Could you check a few things on this drawing? It's one solid part, dimensions in mm from its lowest x, y, z. A direction names the side the tool comes from. Coordinates: 2 decimals unless noted, no trailing zeros. Order: outer loops, then holes, each group sorted by start corner. A loop starts at its lowest first (then second) coordinate and runs counter-clockwise, first axis right, second up. Notation, with made-up numbers: (-34.5, 77.5) - (10.5, 77.5) arc R26 cw to (10.5, 100.5) - close; hole circle Ø1 at (46, 26.5). An arc over 180 degrees is marked (long way). Answer in a Markdown table with one row per item. Add a question column.
Item 1: I want a section at D-D (y = 9). Count the separate pieces of the cut face and the enclosed holes in it.
Item 2: On a 3-axis mill with a long thin cutter (end or side, diameter ignored), from which of +Z, -Z, +X, -X, +Y, -Y can I reach the whole of each face in a straight line? I mean the marked faces 4 and 5. Say none if no direction works.
Item 3: I want a section at B-B (x = 15.5). Please give me the cut outline in (y, z).
Item 4: Will these pins go through, and if not, where does the flat tip stop? pin 1 Ø4 at (x, y) = (7, 9) entering from +Z; pin 2 Ø5 at (y, z) = (12.5, 24) entering from +X; pin 3 Ø5 at (x, z) = (31, 7.5) entering from +Y; pin 4 Ø3 at (y, z) = (2.5, 28) entering from +X.
Item 5: I want a section at C-C (z = 21). Please give me the cut outline in (x, y) (1 decimal).
Item 6: Thinking about a two-plate mould opening in X: for the marked faces 1, 2 and 3, which applies, +X half, -X half, draft (parallel to the pull), parting line (faces both ways), or undercut?
Item 7: I want a section at A-A (z = 7). Please give me the cut outline in (x, y).
Item 8: If I drill on line 1 along Z through (x, y) = (24, 4.5); line 2 along X through (y, z) = (16.5, 13); line 3 along Z through (x, y) = (17.5, 2.5), over which ranges is the centre line in solid material (lowest first)? Write a range as from..to.
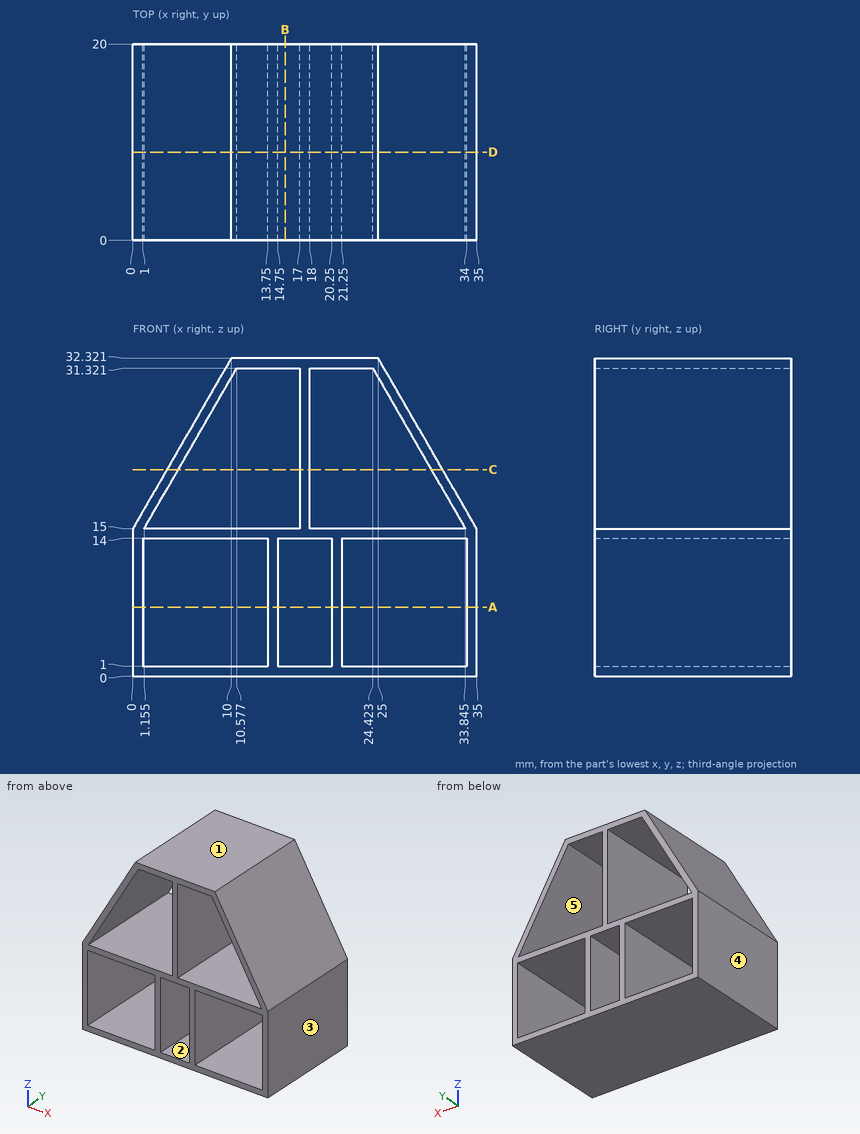
Values follow:
| question | item | result |
|---|---|---|
| 1 | separate pieces | 1 |
| 1 | enclosed holes | 5 |
| 2 | face 4 | +Z, -Z, -X, +Y, -Y |
| 2 | face 5 | +Y, -Y |
| 3 | outline | (0, 0) - (20, 0) - (20, 1) - (0, 1) - close; (0, 14) - (20, 14) - (20, 15) - (0, 15) - close; (0, 31.32) - (20, 31.32) - (20, 32.32) - (0, 32.32) - close |
| 4 | pin 1 | stops at z = 30.59 |
| 4 | pin 2 | stops at x = 31.25 |
| 4 | pin 3 | passes through |
| 4 | pin 4 | stops at x = 28.36 |
| 5 | outline | (3.5, 0) - (4.6, 0) - (4.6, 20) - (3.5, 20) - close; (17, 0) - (18, 0) - (18, 20) - (17, 20) - close; (30.4, 0) - (31.5, 0) - (31.5, 20) - (30.4, 20) - close |
| 6 | face 1 | draft |
| 6 | face 2 | undercut |
| 6 | face 3 | +X half |
| 7 | outline | (0, 0) - (1, 0) - (1, 20) - (0, 20) - close; (13.75, 0) - (14.75, 0) - (14.75, 20) - (13.75, 20) - close; (20.25, 0) - (21.25, 0) - (21.25, 20) - (20.25, 20) - close; (34, 0) - (35, 0) - (35, 20) - (34, 20) - close |
| 8 | line 1 | z = 0..1, 14..15, 31.32..32.32 |
| 8 | line 2 | x = 0..1, 13.75..14.75, 20.25..21.25, 34..35 |
| 8 | line 3 | z = 0..1, 14..32.32 |
